Part model, mm, in its own coordinate system. Give positions to 0.01 mm unless a question says otherwise; leave off trailing zeros. Write each loop counter-clockwise with the first axis right and the second up, starting at its lowest first coordinate (ties: lowest second). Pieces come first, ordered by that corner, then holes. Notation, with made-up numbers: M -37,-27.5 L 22,-27.5 A27 ccw 22,4.5 Z; hole C -20,-31.5 d6. An arc over 180 degrees is marked long. Answer as CSV lines item,"result". Start each with the question number.
Item 1: Band-saw the part on A-A, the plane z = -112.5. List the corners of the cut face in (x, y), then the cut area to 3 significant figures.
Item 2: Wall check: L1, parallel to X at y = -46.5, z = -5.5; L2, parallel to Z at x = 33, y = -43.5 (3 decimals); L3, parallel to Y at x = 40, z = -42. Give the ranges that are in metal, low to high. Write a range as from..to.
Item 3: Band-saw the part on D-D, the plane y = -11.5. List the corners of the cut face in (x, z), then the cut area to 3 significant figures.
Item 4: Pin check, flat tips, straight feed: pin 1 (1 mm diameter, centred on x = -25.5, z = -100.5, fed in from -Y); pin 2 (2 mm diameter, centred on y = -9, z = -27.5, fed in from +X); pin 3 (8 mm diameter, centred on y = -4.5, z = -15.5, fed in from +X). Stop position of each tip, or through.
Item 5: Band-saw the part on C-C, the plane x = -36.5. List the corners of the cut face in (y, z).
Item 6: Band-saw the part on B-B, the plane z = -59. List the corners of the cut face in (x, y).
Autodesk Inventor part; units mm, degrees
ref_plane "YZ Plane" through (0, 0, 0) normal (1, 0, 0) x (0, 1, 0)
ref_plane "XZ Plane" through (0, 0, 0) normal (0, 1, 0) x (-1, 0, 0)
ref_plane "XY Plane" through (0, 0, 0) normal (0, 0, 1) x (1, 0, 0)
sketch "Sketch1" plane through (0, 0, 0) normal (0, 0, 1) x (1, 0, 0)
  line L0 (-44.9013, 44.9013) -> (44.9013, -44.9013)
  line L1 (-44.9013, 44.9013) -> (82.0987, 44.9013) construction
  line L2 (-44.9013, 44.9013) -> (-44.9013, 38.5513)
  line L3 (44.9013, -44.9013) -> (44.9013, -57.6013)
  line L4 (44.9013, -57.6013) -> (-44.9013, 38.5513)
  line L5 (-44.9013, 38.5513) -> (-44.9013, -83.0013) construction
  line L6 (-44.9013, 38.5513) -> (76.6513, 38.5513) construction
  line L7 (44.9013, -57.6013) -> (80.8223, -57.6013) construction
  line L8 (44.9013, -57.6013) -> (37.9664, -50.1761) construction
  line L9 (37.9664, -50.1761) -> (84.3883, -50.1761) construction
  point P0 (0, 0)
  point P1 (0, 0)
  dimension "d0" = 127
  dimension "d1" = 45
  dimension "d2" = 6.35
  dimension "d5" = 12.7
  dimension "d6" = 90
  dimension "d10" = 10.16
extrude "Extrusion1" add sketch "Sketch1" against normal blind 127
sketch "Sketch4" plane through (37.9664, -50.1761, -101.6) normal (-0.7308, -0.6826, 0) x (0, 0, 1)
  line L0 (0, -1.5843) -> (0, 0)
  line L1 (101.6, 0) -> (101.6, -1.5843)
  line L2 (28.575, 11.43) -> (47.625, 11.43)
  line L3 (47.625, 11.43) -> (47.625, 5.08)
  line L4 (47.625, 5.08) -> (28.575, 5.08)
  line L5 (28.575, 5.08) -> (28.575, 11.43)
  line L6 (101.6, 0) -> (-25.4, 0) construction
  line L7 (-25.4, 126.0475) -> (-25.4, -0.8785)
  point P0 (101.6, 62.5845)
  point P1 (38.1, 5.08)
  point P2 (38.1, 0)
  dimension "d24" = 19.05
  dimension "d25" = 6.35
  dimension "d34" = 5.08
extrude "Extrusion4" cut sketch "Sketch4" against normal up to next
sketch "Sketch5" plane through (0, 0, 0) normal (0, 0, 1) x (1, 0, 0)
  line L0 (44.9013, -57.6013) -> (37.9664, -50.1761) construction
  line L1 (44.9013, -57.6013) -> (-44.9013, 38.5513)
  line L2 (32.1524, -62.5572) -> (41.4339, -53.8887) construction
  line L3 (40.1336, -52.4965) -> (42.7341, -55.2809)
  line L4 (29.9852, -60.2368) -> (34.3195, -64.8776)
  line L5 (29.9852, -60.2368) -> (40.1336, -52.4965)
  line L6 (34.3195, -64.8776) -> (42.7341, -55.2809)
  point P0 (0, 0)
  dimension "d28" = 10.16
  dimension "d29" = 12.7
  dimension "d30" = 3.81
  dimension "d31" = 6.35
extrude "Extrusion5" add sketch "Sketch5" against normal blind 114.3
properties part number "proto_1_panel"
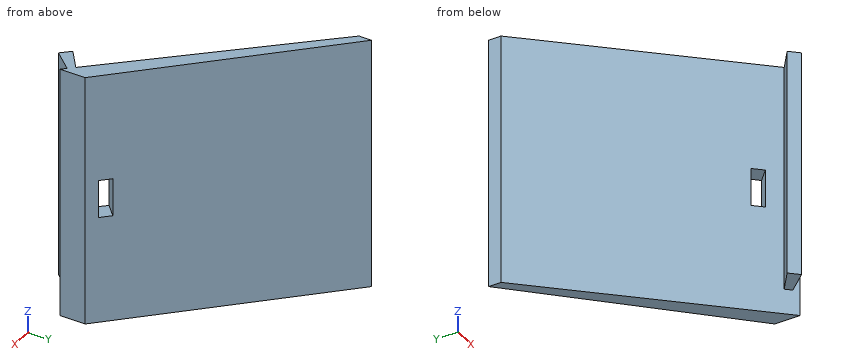
Output:
1,outline,"M -44.9,38.55 L 40.13,-52.5 L 29.99,-60.24 L 34.32,-64.88 L 42.73,-55.28 L 44.9,-57.6 L 44.9,-44.9 L -44.9,44.9 Z"
1,area,"920 mm²"
2,L1,"34.53..44.9"
2,L2,"-127..-73.025, -53.975..0"
2,L3,"-58.4..-52.6, -52.35..-40"
3,outline,"M 1.84,-127 L 11.5,-127 L 11.5,0 L 1.84,0 Z"
3,area,"1,230 mm²"
4,pin 1,"y = 17.24"
4,pin 2,"x = 10"
4,pin 3,"x = 8.5"
5,outline,"M 29.56,-127 L 36.5,-127 L 36.5,0 L 29.56,0 Z"
6,outline,"M -44.9,38.55 L 30.16,-41.82 L 36.19,-36.19 L -44.9,44.9 Z; M 29.99,-60.24 L 34.32,-64.88 L 42.73,-55.28 L 44.9,-57.6 L 44.9,-44.9 L 40.69,-40.69 L 34.5,-46.46 L 40.13,-52.5 Z"
